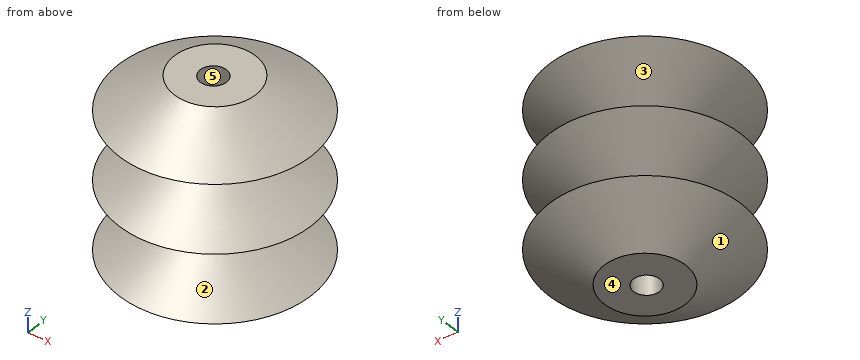
```python
from build123d import *

# Parameters (mm, degrees)
TALADRO_DE_MARGEN_PARA_M81_D = 9


with BuildPart() as part:
    # Croquis1 → Revolución1 (revolve)
    with BuildSketch(Plane(origin=(0, 0, 0), x_dir=(1, 0, 0), z_dir=(0, 1, 0))):
        Polygon((0, 35.444139638), (0, -35.444139638), (14, -35.444139638), (33.031482218, -23.629426425), (14, -11.814713213), (33.031482218, 0), (14, 11.814713213), (33.031482218, 23.629426425), (14, 35.444139638), align=None)
    revolve(axis=Axis((0, 0, -35.444139638), (0, 0, 1)))

    # Taladro de margen para M81 (through all)
    with Locations(Plane.XY.offset(35.444139638)):
        with Locations((-0.173045489, -0.475875094)):
            Hole(TALADRO_DE_MARGEN_PARA_M81_D / 2)


solid = part.part
```
Read the model definition and answer for the solid it produces. Units are mm, in the model's axes. Face numbers are marked on the shaded views. A direction names the side the tool comes from. Coordinates: 2 decimals unless noted, no trailing zeros. Order: outer loops, then holes, each group sorted by start corner. A loop starts at its lowest first (then second) coordinate and runs counter-clockwise, first axis right, second up. Notation, with made-up numbers: (46, 0) - (82, 0) arc R29 ccw to (82, 27) - close; hole circle Ø4 at (9, 87). An arc over 180 degrees is marked (long way). Answer as a JSON object with one key per item and string values. Group by question number.
Item 1: Flat-ended cylindrical pins translate along their axes: P1, Ø3, axis at x = 12, z = 9, coming from the -Y side; P2, Ø8, axis at y = 26.5, z = 24.5, coming from the +X side; P3, Ø6, axis at y = -2, z = 18, coming from the +X side. Find the tip coordinate at first contact, or state that the pin passes through.
Item 2: Consider probe 1 along Z at (x, y) = (16, -25); probe 2 along Z at (x, y) = (18.5, 11.5); probe 3 along X at (y, z) = (3, -10). Determine where each line is inside the solid, lowest interval first. Write a range as from..to.
Item 3: The mould has two halves that part along Y. Classify the marked faces 3, 4 and 5: +Y half, -Y half, draft (parallel to the pull), parting line (faces both ways), or undercut.
Item 4: A tool of negligible diameter and unlimited length cuts with its end or side. For the marked faces 1 and 2, from which of +Z, -Z, +X, -X, +Y, -Y can it reach the whole face along a straight path? Write none if from no direction.
Item 5: Section B-B (z = 9) is taken. Give the vertices of the cut face in (x, y), plus the area to 3 significant figures.
Item 6: Section C-C (y = -22.5) is taken. State how many separate pieces and enclosed holes the cut face has, plus the area to 3 significant figures.
Item 7: Section A-A (x = 0) is taken. Give the vertices of the cut face in (y, z).
Results are:
{
 "1": {"P1": "stops at y = -17.35", "P2": "stops at x = 24.09", "P3": "stops at x = 28.73"},
 "2": {"probe 1": "z = -25.71..-21.55, -2.08..2.08, 21.55..25.71", "probe 2": "z = -30.61..-16.65, -6.98..6.98, 16.65..30.61", "probe 3": "x = -16.66..-3.03, 2.68..16.66"},
 "3": {"face 3": "parting line", "face 4": "draft", "face 5": "undercut"},
 "4": {"face 1": "-Z", "face 2": "none"},
 "5": {"outline": "circle Ø37.07 at (0, 0); hole circle Ø9 at (-0.17, -0.48)", "area": "1,020 mm^2"},
 "6": {"separate pieces": "3", "enclosed holes": "0", "area": "1,220 mm^2"},
 "7": {"outline": "(-33.03, -23.63) - (-14, -35.44) - (-4.97, -35.44) - (-4.97, 35.44) - (-14, 35.44) - (-33.03, 23.63) - (-14, 11.81) - (-33.03, 0) - (-14, -11.81) - close; (4.02, -35.44) - (14, -35.44) - (33.03, -23.63) - (14, -11.81) - (33.03, 0) - (14, 11.81) - (33.03, 23.63) - (14, 35.44) - (4.02, 35.44) - close"}
}
